Can you work these out from the model? Positions are in its coordinate system, mm. Give positions to 0.01 mm unless a question says otherwise; leave off trailing zeros. Order: outer loops, then holes, each group sorted by start corner. A loop starts at its lowest first (then second) coordinate and runs counter-clockwise, first axis right, second up. Notation, with made-up numbers: M 83,79.25 L 119,79.25 A30 cw 119,104.25 Z; hole C 59.25,19 d1. An arc over 180 degrees is marked long. Answer as a JSON object with one key per item and string values.
```python
from build123d import *

# Parameters (mm, degrees)
BOSS_EXTRUDE1_DEPTH = 0.5


with BuildPart() as part:
    # Sketch1 → Boss-Extrude1 (new body)
    with BuildSketch(Plane(origin=(0, 0, 0), x_dir=(1, 0, 0), z_dir=(0, 1, 0))):
        with BuildLine():
            Line((-5.5, 5.5), (-5.5, 4.5))
            ThreePointArc((-5.5, 4.5), (-4.5, 3.5), (-5.5, 2.5))
            Line((-5.5, 2.5), (-5.5, -5.5))
            Line((-5.5, -5.5), (-2.5, -5.5))
            Line((-2.5, -5.5), (-2.5, 0))
            ThreePointArc((-2.5, 0), (0, 2.5), (2.5, 0))
            Line((2.5, 0), (2.5, -5.5))
            Line((2.5, -5.5), (5.5, -5.5))
            Line((5.5, -5.5), (5.5, 2.5))
            ThreePointArc((5.5, 2.5), (4.5, 3.5), (5.5, 4.5))
            Line((5.5, 4.5), (5.5, 5.5))
            Line((5.5, 5.5), (-5.5, 5.5))
        make_face()
    extrude(amount=BOSS_EXTRUDE1_DEPTH)


solid = part.part
```
1) I want a section at C-C on x = 0. Write out the boundary of the cut face in (y, z), and give its area (3 significant figures).
Results found:
{"outline": "M 0,-5.5 L 0.5,-5.5 L 0.5,-2.5 L 0,-2.5 Z", "area": "1.50 mm²"}
2) I want a section at A-A on z = -2. Write out the boundary of the cut face in (x, y), and give its area (3 significant figures).
Results found:
{"outline": "M -5.5,0 L -1.5,0 L -1.5,0.5 L -5.5,0.5 Z; M 1.5,0 L 5.5,0 L 5.5,0.5 L 1.5,0.5 Z", "area": "4.00 mm²"}
3) I want a section at D-D on z = 2.25. Write out the boundary of the cut face in (x, y).
Results found:
{"outline": "M -5.5,0 L -2.5,0 L -2.5,0.5 L -5.5,0.5 Z; M 2.5,0 L 5.5,0 L 5.5,0.5 L 2.5,0.5 Z"}
4) Thinking about a two-plate mould opening in X: for faces 1 (the face through (-0.1, 0.2, -2.5)), 2 (the face through (4.5, 0.2, -3.5)), 3 (the face through (0, 0.5, -3)), 4 (the face through (-4.5, 0.2, -3.5)), which applies, pulls with the +X half, pulls with the -X half, needs draft (parallel to the pull), parting line crosses it, or undercut?
Results found:
{"face 1": "undercut", "face 2": "pulls with the +X half", "face 3": "needs draft", "face 4": "pulls with the -X half"}
5) I need wall thicknesses on L1, parallel to X at y = 0.3, z = 3.75; L2, parallel to X at y = 0.2, z = -3.5; L3, parallel to X at y = 0.25, z = -1. Which ranges of each line are inside material? Lowest first, please.
Results found:
{"L1": "x = -5.5 to -2.5, 2.5 to 5.5", "L2": "x = -4.5 to 4.5", "L3": "x = -5.5 to -2.29, 2.29 to 5.5"}
6) I'm going to push a flat-ended pin straight in: pin 1 Ø6 at (x, z) = (2.5, -1.5) entering from -Y. Where does the tip first touch, or does it pass through?
Results found:
{"pin 1": "stops at y = 0"}
7) I want a section at B-B on y = 0.4. Write out the boundary of the cut face in (x, z).
Results found:
{"outline": "M -5.5,-5.5 L 5.5,-5.5 L 5.5,-4.5 A1 cw 5.5,-2.5 L 5.5,5.5 L 2.5,5.5 L 2.5,0 A2.5 cw -2.5,0 L -2.5,5.5 L -5.5,5.5 L -5.5,-2.5 A1 cw -5.5,-4.5 Z"}
